Design review of the part shown in the three views and the two pictorial views. Dimensions are in mm from the part's minimum x, y and z. Round coordinates to 2 decimals unless told otherwise and drop trailing zeros. Loops run counter-clockwise (first coordinate to the right, second up) from the corner with the lowest first, then second, coordinate; pieces in that order, holes last. Notation, with made-up numbers: (75.25, 37) -> (83.25, 37) arc R25 cw to (83.25, 64) -> close; hole circle Ø7 at (-8.75, -25.5). An arc over 180 degrees is marked (long way). One line per question, with ' | ' between items. Start each with the question number.
1. Consider section C-C (y = 27.5). Write out the cut boundary in (x, z), and give its area (3 significant figures).
2. For pin 1 Ø1 at (x, y) = (13.5, 6.5) entering from +Z; pin 2 Ø3 at (y, z) = (28.5, 25) entering from +X; pin 3 Ø10 at (x, y) = (4, 28.5) entering from -Z, all flat-tipped, find the tip position at first contact; note any pin that passes through.
3. Wall thickness on line 1 along Y through (x, z) = (18.5, 28.75); line 2 along Z through (x, y) = (15.75, 21) (1 decimal); line 3 along Z through (x, y) = (3.25, 19.5) (1 decimal): over which ranges is each line inside the solid? List them lowest first.
4. Consider section B-B (x = 26.75). Write out the cut boundary in (y, z) (1 decimal), and give its area (3 significant figures).
5. Consider section A-A (z = 28). Write out the cut boundary in (x, y), and give its area (3 significant figures).
6. Consider section D-D (z = 10.5). Write out the cut boundary in (x, y), and give its area (3 significant figures).
7. Draft analysis for pull direction X (two halves, no side actions). For the marked faces 1, 2 and 3, state which applies: pulls with the +X half, pulls with the -X half, needs draft (parallel to the pull), parting line crosses it, or undercut.
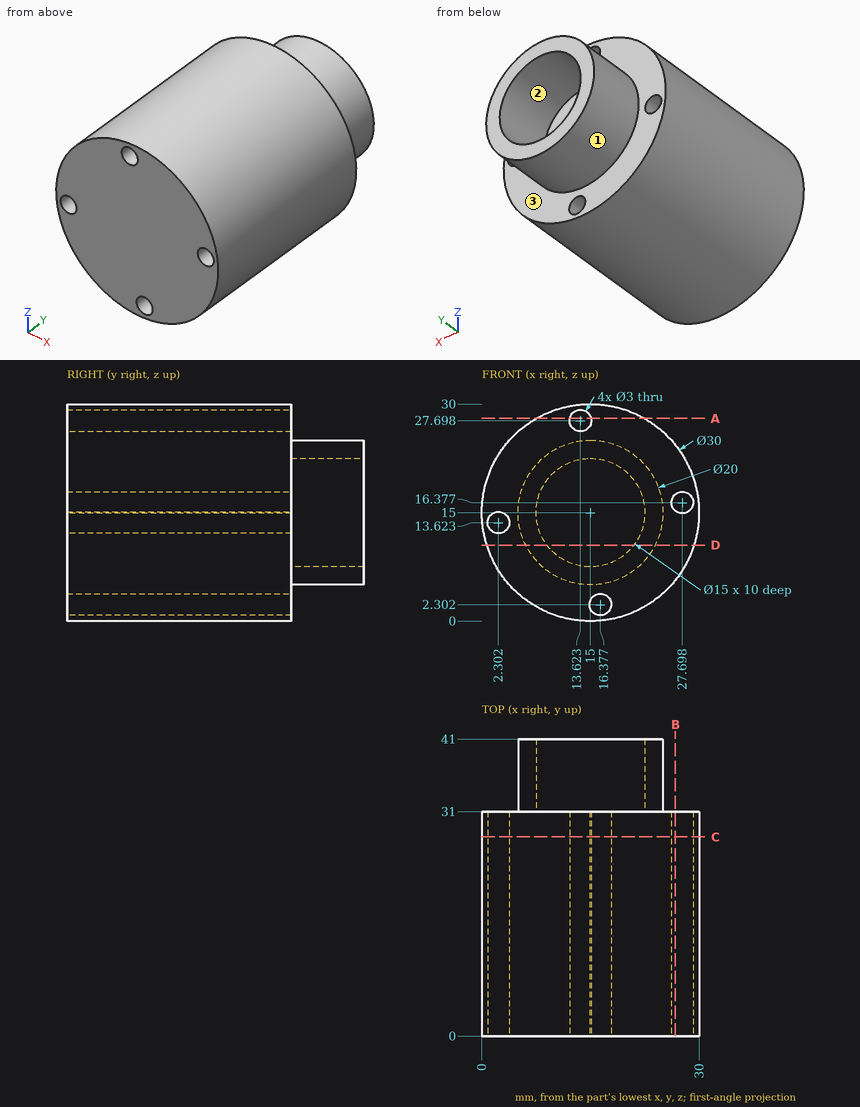
Answer block:
1) outline: circle Ø30 at (15, 15); hole circle Ø3 at (2.3, 13.62); hole circle Ø3 at (13.62, 27.7); hole circle Ø3 at (16.38, 2.3); hole circle Ø3 at (27.7, 16.38) | area: 679 mm2
2) pin 1: stops at z = 29.97 | pin 2: stops at x = 27.36 | pin 3: stops at z = 1.25
3) line 1: y = 0 to 31 | line 2: z = 0 to 0.9, 3.7 to 30 | line 3: z = 5.7 to 12.5, 14.8 to 24.3
4) outline: (0, 5.7) -> (31, 5.7) -> (31, 15.2) -> (0, 15.2) -> close; (0, 17.5) -> (31, 17.5) -> (31, 24.3) -> (0, 24.3) -> close | area: 506 mm2
5) outline: (7.52, 0) -> (12.15, 0) -> (12.15, 31) -> (7.52, 31) -> close; (15.09, 0) -> (22.48, 0) -> (22.48, 31) -> (15.09, 31) -> close | area: 373 mm2
6) outline: (0.69, 0) -> (29.31, 0) -> (29.31, 31) -> (23.93, 31) -> (23.93, 41) -> (21, 41) -> (21, 31) -> (9, 31) -> (9, 41) -> (6.07, 41) -> (6.07, 31) -> (0.69, 31) -> close | area: 946 mm2
7) face 1: parting line crosses it | face 2: undercut | face 3: needs draft
